CAD build for the part. Positions are in the model's coordinates, mm. Face numbers are marked on the shaded views. A direction names the side the tool comes from. Round coordinates to 2 decimals unless told otherwise and drop trailing zeros. Loops run counter-clockwise (first coordinate to the right, second up) from the corner with the lowest first, then second, coordinate; pieces in that order, holes last.
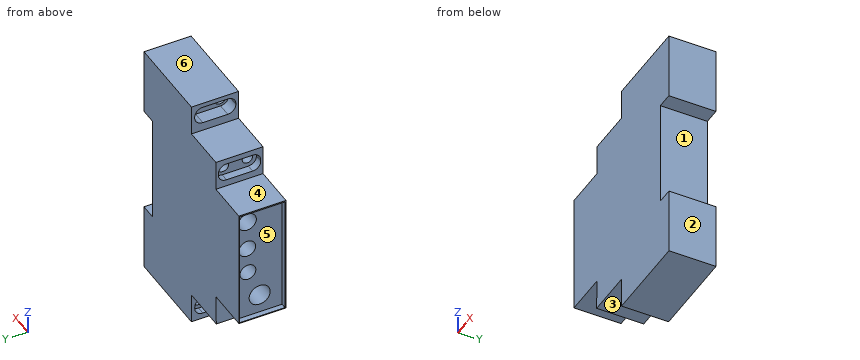
```python
from build123d import *

# Parameters (mm, degrees)
F1_DEPTH  = 17.5
F2_R      = 2.25021
F2_R_2    = 2.117892
F2_R_3    = 2.141219
F2_R_4    = 1.925027
F2_R_5    = 3.371511
F2_R_6    = 3.105781
F2_R_7    = 1.98861
F2_R_8    = 1.899979
F2_R_9    = 1.912547
F3_DEPTH  = 40
F4_R      = 2.117892
F4_R_2    = 2.25021
F5_DEPTH  = 5
F6_R      = 2.141219
F6_R_2    = 1.925027
F7_DEPTH  = 3
F9_DEPTH  = 3
F10_W     = 16.805832
F10_H     = 44.291496
F10_R     = 3.105781
F10_R_2   = 3.371511
F11_DEPTH = 2
F12_R     = 2.950074
F12_R_2   = 3.899051
F13_DEPTH = 25


with BuildPart() as f1:
    # F0 (on Front) → F1 (new body)
    with BuildSketch(Plane.XZ):
        Polygon((-29.036315, 123.591392), (-62.036315, 123.591392), (-62.036315, 112.341392), (-79.036315, 112.341392), (-79.036315, 101.091392), (-95.036315, 101.091392), (-95.036315, 56.091392), (-79.036315, 56.091392), (-79.313149, 44.841392), (-62.036315, 44.841392), (-62.036315, 33.591392), (-29.036315, 33.591392), (-29.036315, 58.591392), (-35.036315, 58.591392), (-35.036315, 98.591392), (-29.036315, 98.591392), align=None)
    extrude(amount=F1_DEPTH)

    # F2 (on face) → F3 (cut)
    with BuildSketch(Plane(origin=(-95.036315, 0, 0), x_dir=(0, -1, 0), z_dir=(-1, 0, 0))):
        with Locations((13.294209, 118.739031)):
            Circle(F2_R)
        with Locations((4.177382, 118.739031)):
            Circle(F2_R_2)
        with Locations((4.177382, 106.985271)):
            Circle(F2_R_3)
        with Locations((13.294209, 106.985271)):
            Circle(F2_R_4)
        with Locations((4.177382, 95.644102)):
            Circle(F2_R_5)
        with Locations((4.177382, 84.471688)):
            Circle(F2_R_6)
        with Locations((4.177382, 39.11674)):
            Circle(F2_R_7)
        with Locations((8.744364, 39.11674)):
            Circle(F2_R_8)
        with Locations((13.294209, 39.11674)):
            Circle(F2_R_9)
    extrude(amount=-F3_DEPTH, mode=Mode.SUBTRACT)

    # F4 (on face) → F5 (cut)
    with BuildSketch(Plane(origin=(-62.036315, 0, 0), x_dir=(0, -1, 0), z_dir=(-1, 0, 0))):
        with BuildLine():
            Line((13.491717, 121.922452), (4.209779, 121.922452))
            ThreePointArc((4.209779, 121.922452), (2.088459, 121.043773), (1.209779, 118.922452))
            Line((1.209779, 118.922452), (1.209779, 118.510082))
            ThreePointArc((1.209779, 118.510082), (2.088459, 116.388762), (4.209779, 115.510082))
            Line((4.209779, 115.510082), (13.491717, 115.510082))
            ThreePointArc((13.491717, 115.510082), (15.613037, 116.388762), (16.491717, 118.510082))
            Line((16.491717, 118.510082), (16.491717, 118.922452))
            ThreePointArc((16.491717, 118.922452), (15.613037, 121.043773), (13.491717, 121.922452))
        make_face()
        with Locations((4.177382, 118.739031)):
            Circle(F4_R, mode=Mode.SUBTRACT)
        with Locations((13.294209, 118.739031)):
            Circle(F4_R_2, mode=Mode.SUBTRACT)
    extrude(amount=-F5_DEPTH, mode=Mode.SUBTRACT)

    # F6 (on face) → F7 (cut)
    with BuildSketch(Plane(origin=(-79.036315, 0, 0), x_dir=(0, -1, 0), z_dir=(-1, 0, 0))):
        with BuildLine():
            Line((13.656557, 110.275699), (3.933159, 110.275699))
            ThreePointArc((3.933159, 110.275699), (1.811838, 109.397019), (0.933159, 107.275699))
            Line((0.933159, 107.275699), (0.933159, 106.589088))
            ThreePointArc((0.933159, 106.589088), (1.811838, 104.467767), (3.933159, 103.589088))
            Line((3.933159, 103.589088), (13.656557, 103.589088))
            ThreePointArc((13.656557, 103.589088), (15.777877, 104.467767), (16.656557, 106.589088))
            Line((16.656557, 106.589088), (16.656557, 107.275699))
            ThreePointArc((16.656557, 107.275699), (15.777877, 109.397019), (13.656557, 110.275699))
        make_face()
        with Locations((4.177382, 106.985271)):
            Circle(F6_R, mode=Mode.SUBTRACT)
        with Locations((13.294209, 106.985271)):
            Circle(F6_R_2, mode=Mode.SUBTRACT)
    extrude(amount=-F7_DEPTH, mode=Mode.SUBTRACT)

    # F8 (on face) → F9 (cut)
    with BuildSketch(Plane(origin=(-62.036315, 0, 0), x_dir=(0, -1, 0), z_dir=(-1, 0, 0))):
        with BuildLine():
            ThreePointArc((1.226484, 38.683788), (2.105164, 36.562468), (4.226484, 35.683788))
            Line((4.226484, 35.683788), (13.570151, 35.683788))
            ThreePointArc((13.570151, 35.683788), (15.691471, 36.562468), (16.570151, 38.683788))
            Line((16.570151, 38.683788), (16.570151, 39.214782))
            ThreePointArc((16.570151, 39.214782), (15.691471, 41.336103), (13.570151, 42.214782))
            Line((13.570151, 42.214782), (4.226484, 42.214782))
            ThreePointArc((4.226484, 42.214782), (2.105164, 41.336103), (1.226484, 39.214782))
            Line((1.226484, 39.214782), (1.226484, 38.683788))
        make_face()
    extrude(amount=-F9_DEPTH, mode=Mode.SUBTRACT)

    # F10 (on face) → F11 (cut)
    with BuildSketch(Plane(origin=(-95.036315, 0, 0), x_dir=(0, -1, 0), z_dir=(-1, 0, 0))):
        with Locations((8.686814, 78.51769)):
            Rectangle(F10_W, F10_H)
        with Locations((4.177382, 84.471688)):
            Circle(F10_R, mode=Mode.SUBTRACT)
        with Locations((4.177382, 95.644102)):
            Circle(F10_R_2, mode=Mode.SUBTRACT)
    extrude(amount=-F11_DEPTH, mode=Mode.SUBTRACT)

    # F12 (on face) → F13 (cut)
    with BuildSketch(Plane(origin=(-93.036315, 0, 0), x_dir=(0, -1, 0), z_dir=(-1, 0, 0))):
        with Locations((4.417871, 74.5501)):
            Circle(F12_R)
        with Locations((8.776497, 63.428089)):
            Circle(F12_R_2)
    extrude(amount=-F13_DEPTH, mode=Mode.SUBTRACT)


solid = f1.part
```
Item 1: Cut at A-A, the plane z = 79.5. Give the cut face in (x, y).
Answers follow:
outline: (-95.04, -17.5) - (-35.04, -17.5) - (-35.04, 0) - (-95.04, 0) - (-95.04, -0.28) - (-93.04, -0.28) - (-93.04, -17.09) - (-95.04, -17.09) - close
Item 2: Flat gauge pins, fed straight in: P1, Ø5, axis at y = -9, z = 92.5, coming from the -X side; P2, Ø2, axis at y = -5.5, z = 40, coming from the -X side; P3, Ø2, axis at x = -63.5, y = -11, coming from the +Z side. Where does each tip first touch, or does it go through?
Answers follow:
P1: stops at x = -93.04
P2: stops at x = -59.04
P3: stops at z = 112.34
Item 3: 3-axis set-ups, long thin cutter, end or side, ignore diameter. For the marked faces 4, 5 and 6: which of +Z, -Z, +X, -X, +Y, -Y reach the whole face in a straight line?
Answers follow:
face 4: +Z, -X, +Y, -Y
face 5: -X
face 6: +Z, +X, -X, +Y, -Y
Item 4: Probe line 1 (Z direction, x = -62, y = -6); line 2 (Z direction, x = -73.5, y = -9); line 3 (Z direction, x = -57, y = -2.5). List the from-to ranges inside material, lowest first.
Answers follow:
line 1: z = 33.59 to 35.68, 42.21 to 81.96, 86.99 to 92.81, 98.48 to 105.86, 108.11 to 115.51, 121.92 to 123.59
line 2: z = 44.84 to 59.54, 67.32 to 112.34
line 3: z = 33.59 to 38.05, 40.18 to 81.86, 87.09 to 92.72, 98.57 to 105.65, 108.32 to 117.45, 120.03 to 123.59
Item 5: Cut at D-D, the plane x = -77. Give the cut face in (y, z).
Answers follow:
outline: (-17.5, 44.84) - (0, 44.84) - (0, 112.34) - (-17.5, 112.34) - close; hole (-16.66, 106.59) arc R3 ccw to (-13.66, 103.59) - (-3.93, 103.59) arc R3 ccw to (-0.93, 106.59) - (-0.93, 107.28) arc R3 ccw to (-3.93, 110.28) - (-13.66, 110.28) arc R3 ccw to (-16.66, 107.28) - close; hole circle Ø7.8 at (-8.78, 63.43); hole circle Ø6.74 at (-4.18, 95.64); hole circle Ø5.9 at (-4.42, 74.55); hole circle Ø6.21 at (-4.18, 84.47)
Item 6: Cut at C-C, the plane x = -70. Give the cut face in (y, z).
Answers follow:
outline: (-17.5, 44.84) - (0, 44.84) - (0, 112.34) - (-17.5, 112.34) - close; hole circle Ø3.85 at (-13.29, 106.99); hole circle Ø7.8 at (-8.78, 63.43); hole circle Ø6.74 at (-4.18, 95.64); hole circle Ø5.9 at (-4.42, 74.55); hole circle Ø6.21 at (-4.18, 84.47); hole circle Ø4.28 at (-4.18, 106.99)
Item 7: Two-plate mould, pull along Z, no slides. Class the marked faces 1, 2 and 3: released by +Z, released by -Z, zero draft, split by the parting line, or undercut.
Answers follow:
face 1: undercut
face 2: zero draft
face 3: released by -Z
Item 8: Cut at B-B, the plane x = -89.5. Give the cut face in (y, z), plus the area to 3 significant figures.
Answers follow:
outline: (-17.5, 56.09) - (0, 56.09) - (0, 101.09) - (-17.5, 101.09) - close; hole circle Ø7.8 at (-8.78, 63.43); hole circle Ø6.74 at (-4.18, 95.64); hole circle Ø5.9 at (-4.42, 74.55); hole circle Ø6.21 at (-4.18, 84.47)
area: 646 mm2
